Work out the finished part from the listing and answer in its coordinate system (mm). Face numbers are marked on the shaded views. A direction names the side the tool comes from. Give positions to 0.01 mm unless a question says otherwise; leave off trailing zeros. Order: outer loops, then holes, each group sorted by start corner. A loop starts at its lowest first (then second) coordinate and runs counter-clockwise, first axis right, second up.
```python
from build123d import *

# Parameters (mm, degrees)
SKETCH1_W           = 76.2
SKETCH1_H           = 57.15
BOSS_EXTRUDE1_DEPTH = 6.35


with BuildPart() as part:
    # Sketch1 → Boss-Extrude1 (new, symmetric)
    with BuildSketch(Plane(origin=(0, 0, 0), x_dir=(1, 0, 0), z_dir=(0, 1, 0))):
        Rectangle(SKETCH1_W, SKETCH1_H)
        with BuildLine():
            Line((-25.4, 6.985), (25.4, 6.985))
            ThreePointArc((25.4, 6.985), (32.385, 0), (25.4, -6.985))
            Line((25.4, -6.985), (-25.4, -6.985))
            ThreePointArc((-25.4, -6.985), (-32.385, 0), (-25.4, 6.985))
        make_face(mode=Mode.SUBTRACT)
    extrude(amount=BOSS_EXTRUDE1_DEPTH, both=True)


solid = part.part
```
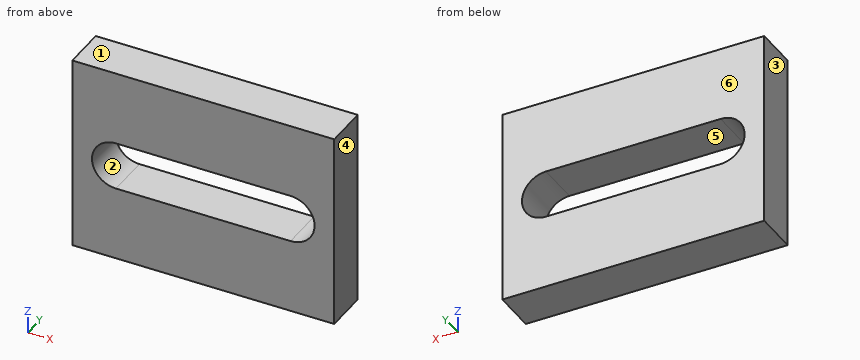
1. The part is cut by section B-B (y = 0.5). Write down the section's boundary in (x, z) (3 decimals), then the cut area to 3 significant figures.
Findings below:
outline: (-38.1, -28.575) - (38.1, -28.575) - (38.1, 28.575) - (-38.1, 28.575) - close; hole (-25.4, -6.985) - (25.4, -6.985) arc R6.985 ccw to (25.4, 6.985) - (-25.4, 6.985) arc R6.985 ccw to start
area: 3,490 mm2
2. Straight lines are drawn through the part: probe 1 along Z at (x, y) = (-13, 4) (3 decimals); probe 2 along X at (y, z) = (-2, -0.5); probe 3 along Z at (x, y) = (31.5, -5) (3 decimals). For each, find the intervals that lie inside material, in ascending order.
Findings below:
probe 1: z = -28.575 to -6.985, 6.985 to 28.575
probe 2: x = -38.1 to -32.37, 32.37 to 38.1
probe 3: z = -28.575 to -3.403, 3.403 to 28.575
3. The mould has two halves that part along X. Classify the marked faces 3, 4, 5 and 6: pulls with the +X half, pulls with the -X half, needs draft (parallel to the pull), parting line crosses it, or undercut.
Findings below:
face 3: pulls with the -X half
face 4: pulls with the +X half
face 5: undercut
face 6: needs draft
4. Which of the six approach directions +Z, -Z, +X, -X, +Y, -Y give full straight-line access (tool end or side, diameter ignored) to the marked faces 1 and 2?
Findings below:
face 1: +Z, +X, -X, +Y, -Y
face 2: +Y, -Y
5. The part is cut by section A-A (z = 0). Write down the section's boundary in (x, y) (3 decimals), then the cut area to 3 significant figures.
Findings below:
outline: (-38.1, -6.35) - (-32.385, -6.35) - (-32.385, 6.35) - (-38.1, 6.35) - close; (32.385, -6.35) - (38.1, -6.35) - (38.1, 6.35) - (32.385, 6.35) - close
area: 145 mm2
6. The part is cut by section C-C (x = 12). Write down the section's boundary in (y, z) (3 decimals).
Findings below:
outline: (-6.35, -28.575) - (6.35, -28.575) - (6.35, -6.985) - (-6.35, -6.985) - close; (-6.35, 6.985) - (6.35, 6.985) - (6.35, 28.575) - (-6.35, 28.575) - close
